```python
from build123d import *

# Parameters (mm, degrees)
F0_W          = 20
F0_H          = 20
F1_DEPTH      = 20
F3_R          = 2
F8_DEPTH      = 1
F2_R          = 2
F11_DEPTH     = 1
F6_R          = 2.787917168
F12_DEPTH     = 1
F4_R          = 2
F13_DEPTH     = 1
F14_DEPTH     = 1
F5_R          = 2
F15_DEPTH     = 1
F7_R          = 2
F16_DEPTH     = 1
F17_T1_DEPTH  = 16
F17_T3_DEPTH  = 16
F17_T5_DEPTH  = 16
F17_S9_W      = 2
F17_S9_H      = 2
F17_T10_DEPTH = 2
F17_S15_W     = 2
F17_S15_H     = 2
F17_T16_DEPTH = 2
F17_S21_W     = 2
F17_S21_H     = 2
F17_T22_DEPTH = 2
F17_S27_W     = 2
F17_S27_H     = 2
F17_T28_DEPTH = 2
F17_S33_W     = 2
F17_S33_H     = 2
F17_T34_DEPTH = 2
F17_S39_W     = 2
F17_S39_H     = 2
F17_T40_DEPTH = 2
F17_S45_W     = 2
F17_S45_H     = 2
F17_T46_DEPTH = 2
F17_S51_W     = 2
F17_S51_H     = 2
F17_T52_DEPTH = 2


# Not quite as in the source:
# - a fillet or chamfer that OpenCascade refuses, or shapes differently, is made with other operations: its cross-section is extruded or revolved along the edge and cut away or added
# - a feature of the source that left no trace in its solid (it failed there, or was rolled back) is left out


with BuildPart() as f1:
    # F0 (on Top) → F1 (new body)
    with BuildSketch(Plane.XY):
        with Locations((10, 10)):
            Rectangle(F0_W, F0_H)
    extrude(amount=F1_DEPTH)

    # F3 (on face) → F8 (cut)
    with BuildSketch(Plane.XY.offset(20)):
        with Locations((4.0282921307, 15.9717078693)):
            Circle(F3_R)
        with Locations((4.0282921307, 9.9717078693)):
            Circle(F3_R)
        with Locations((4.0282921307, 3.9717078693)):
            Circle(F3_R)
        with Locations((16.0282921307, 15.9717078693)):
            Circle(F3_R)
        with Locations((16.0282921307, 9.9717078693)):
            Circle(F3_R)
        with Locations((16.0282921307, 3.9717078693)):
            Circle(F3_R)
    extrude(amount=-F8_DEPTH, mode=Mode.SUBTRACT)

    # F2 (on Top) → F11 (cut)
    with BuildSketch(Plane.XY):
        with Locations((10, 10)):
            Circle(F2_R)
    extrude(amount=F11_DEPTH, mode=Mode.SUBTRACT)

    # F6 (on face) → F12 (cut)
    with BuildSketch(Plane(origin=(0, 0, 0), x_dir=(0, -1, 0), z_dir=(-1, 0, 0))):
        with Locations((-15.4005342424, 15.4005342424)):
            Circle(F6_R)
        with Locations((-10.667038206, 10.667038206)):
            Circle(F6_R)
        with Locations((-5.3520903582, 5.3520903582)):
            Circle(F6_R)
    extrude(amount=-F12_DEPTH, mode=Mode.SUBTRACT)

    # F4 (on Front) → F13 (cut)
    with BuildSketch(Plane.XZ):
        with Locations((16, 4)):
            Circle(F4_R)
        with Locations((4, 16)):
            Circle(F4_R)
        with Locations((16, 16)):
            Circle(F4_R)
        with Locations((4, 4)):
            Circle(F4_R)
        with Locations((10, 10)):
            Circle(F4_R)
    extrude(amount=-F13_DEPTH, mode=Mode.SUBTRACT)

    # F6 (on face) → F14 (cut)
    with BuildSketch(Plane(origin=(0, 0, 0), x_dir=(0, -1, 0), z_dir=(-1, 0, 0))):
        with Locations((-15.4005342424, 15.4005342424)):
            Circle(F6_R)
        with Locations((-10.667038206, 10.667038206)):
            Circle(F6_R)
        with Locations((-5.3520903582, 5.3520903582)):
            Circle(F6_R)
    extrude(amount=-F14_DEPTH, mode=Mode.SUBTRACT)

    # F5 (on face) → F15 (cut)
    with BuildSketch(Plane(origin=(0, 20, 0), x_dir=(-1, 0, 0), z_dir=(0, 1, 0))):
        with Locations((-13.3333333333, 13.3333333333)):
            Circle(F5_R)
        with Locations((-6.6666666667, 6.6666666667)):
            Circle(F5_R)
    extrude(amount=-F15_DEPTH, mode=Mode.SUBTRACT)

    # F7 (on face) → F16 (cut)
    with BuildSketch(Plane.YZ.offset(20)):
        with Locations((16, 4)):
            Circle(F7_R)
        with Locations((16, 16)):
            Circle(F7_R)
        with Locations((4, 16)):
            Circle(F7_R)
        with Locations((4, 4)):
            Circle(F7_R)
    extrude(amount=-F16_DEPTH, mode=Mode.SUBTRACT)

    # F17: fillet of radius 2 on 12 edges, made by hand

    # F17_s2 → F17_t1 (cut)
    with BuildSketch(Plane.YZ.offset(2)):
        with BuildLine():
            ThreePointArc((20, 2), (19.4142135624, 0.5857864376), (18, 0))
            Line((18, 0), (20, 0))
            Line((20, 0), (20, 2))
        make_face()
        with BuildLine():
            ThreePointArc((2, 0), (0.5857864376, 0.5857864376), (0, 2))
            Line((0, 2), (0, 0))
            Line((0, 0), (2, 0))
        make_face()
        with BuildLine():
            ThreePointArc((2, 20), (0.5857864376, 19.4142135624), (0, 18))
            Line((0, 18), (0, 20))
            Line((0, 20), (2, 20))
        make_face()
        with BuildLine():
            ThreePointArc((20, 18), (19.4142135624, 19.4142135624), (18, 20))
            Line((18, 20), (20, 20))
            Line((20, 20), (20, 18))
        make_face()
    extrude(amount=F17_T1_DEPTH, mode=Mode.SUBTRACT)

    # F17_s4 → F17_t3 (cut)
    with BuildSketch(Plane.XZ.offset(-18)):
        with BuildLine():
            ThreePointArc((18, 0), (19.4142135624, 0.5857864376), (20, 2))
            Line((20, 2), (20, 0))
            Line((20, 0), (18, 0))
        make_face()
        with BuildLine():
            ThreePointArc((0, 2), (0.5857864376, 0.5857864376), (2, 0))
            Line((2, 0), (0, 0))
            Line((0, 0), (0, 2))
        make_face()
        with BuildLine():
            ThreePointArc((0, 18), (0.5857864376, 19.4142135624), (2, 20))
            Line((2, 20), (0, 20))
            Line((0, 20), (0, 18))
        make_face()
        with BuildLine():
            ThreePointArc((18, 20), (19.4142135624, 19.4142135624), (20, 18))
            Line((20, 18), (20, 20))
            Line((20, 20), (18, 20))
        make_face()
    extrude(amount=F17_T3_DEPTH, mode=Mode.SUBTRACT)

    # F17_s6 → F17_t5 (cut)
    with BuildSketch(Plane.XY.offset(2)):
        with BuildLine():
            ThreePointArc((0, 2), (0.5857864376, 0.5857864376), (2, 0))
            Line((2, 0), (0, 0))
            Line((0, 0), (0, 2))
        make_face()
        with BuildLine():
            ThreePointArc((0, 18), (0.5857864376, 19.4142135624), (2, 20))
            Line((2, 20), (0, 20))
            Line((0, 20), (0, 18))
        make_face()
        with BuildLine():
            ThreePointArc((18, 0), (19.4142135624, 0.5857864376), (20, 2))
            Line((20, 2), (20, 0))
            Line((20, 0), (18, 0))
        make_face()
        with BuildLine():
            ThreePointArc((18, 20), (19.4142135624, 19.4142135624), (20, 18))
            Line((20, 18), (20, 20))
            Line((20, 20), (18, 20))
        make_face()
    extrude(amount=F17_T5_DEPTH, mode=Mode.SUBTRACT)


with BuildPart() as f17_tool8:
    # F17_s9 → F17_t10 (new body)
    with BuildSketch(Plane.YZ.offset(18)):
        with Locations((19, 1)):
            Rectangle(F17_S9_W, F17_S9_H)
    extrude(amount=F17_T10_DEPTH)

    # F17_s11 → F17_t12 (revolve, cut)
    with BuildSketch(Plane(origin=(18, 18, 2), x_dir=(0, -0.7071067812, 0.7071067812), z_dir=(0, 0.7071067812, 0.7071067812))):
        with BuildLine():
            ThreePointArc((0, -2), (2, 0), (0, 2))
            Line((0, 2), (0, -2))
        make_face()
    revolve(axis=Axis((18, 18, 2), (1, 0, 0)), mode=Mode.SUBTRACT)


with BuildPart() as f1_1:
    add(f1.part)

    # F17_t7: cut F17_tool8
    add(f17_tool8.part, mode=Mode.SUBTRACT)


with BuildPart() as f17_tool14:
    # F17_s15 → F17_t16 (new body)
    with BuildSketch(Plane.YZ.offset(2)):
        with Locations((19, 1)):
            Rectangle(F17_S15_W, F17_S15_H)
    extrude(amount=-F17_T16_DEPTH)

    # F17_s17 → F17_t18 (revolve, cut)
    with BuildSketch(Plane(origin=(2, 18, 2), x_dir=(0, -0.7071067812, 0.7071067812), z_dir=(0, -0.7071067812, -0.7071067812))):
        with BuildLine():
            ThreePointArc((0, -2), (2, 0), (0, 2))
            Line((0, 2), (0, -2))
        make_face()
    revolve(axis=Axis((2, 18, 2), (-1, 0, 0)), mode=Mode.SUBTRACT)


with BuildPart() as f1_2:
    add(f1_1.part)

    # F17_t13: cut F17_tool14
    add(f17_tool14.part, mode=Mode.SUBTRACT)


with BuildPart() as f17_tool20:
    # F17_s21 → F17_t22 (new body)
    with BuildSketch(Plane.YZ.offset(18)):
        with Locations((1, 1)):
            Rectangle(F17_S21_W, F17_S21_H)
    extrude(amount=F17_T22_DEPTH)

    # F17_s23 → F17_t24 (revolve, cut)
    with BuildSketch(Plane(origin=(18, 2, 2), x_dir=(0, 0.7071067812, 0.7071067812), z_dir=(0, 0.7071067812, -0.7071067812))):
        with BuildLine():
            ThreePointArc((0, -2), (2, 0), (0, 2))
            Line((0, 2), (0, -2))
        make_face()
    revolve(axis=Axis((18, 2, 2), (1, 0, 0)), mode=Mode.SUBTRACT)


with BuildPart() as f1_3:
    add(f1_2.part)

    # F17_t19: cut F17_tool20
    add(f17_tool20.part, mode=Mode.SUBTRACT)


with BuildPart() as f17_tool26:
    # F17_s27 → F17_t28 (new body)
    with BuildSketch(Plane.YZ.offset(2)):
        with Locations((1, 1)):
            Rectangle(F17_S27_W, F17_S27_H)
    extrude(amount=-F17_T28_DEPTH)

    # F17_s29 → F17_t30 (revolve, cut)
    with BuildSketch(Plane(origin=(2, 2, 2), x_dir=(0, 0.7071067812, 0.7071067812), z_dir=(0, -0.7071067812, 0.7071067812))):
        with BuildLine():
            ThreePointArc((0, -2), (2, 0), (0, 2))
            Line((0, 2), (0, -2))
        make_face()
    revolve(axis=Axis((2, 2, 2), (-1, 0, 0)), mode=Mode.SUBTRACT)


with BuildPart() as f1_4:
    add(f1_3.part)

    # F17_t25: cut F17_tool26
    add(f17_tool26.part, mode=Mode.SUBTRACT)


with BuildPart() as f17_tool32:
    # F17_s33 → F17_t34 (new body)
    with BuildSketch(Plane.YZ.offset(2)):
        with Locations((1, 19)):
            Rectangle(F17_S33_W, F17_S33_H)
    extrude(amount=-F17_T34_DEPTH)

    # F17_s35 → F17_t36 (revolve, cut)
    with BuildSketch(Plane(origin=(2, 2, 18), x_dir=(0, 0.7071067812, -0.7071067812), z_dir=(0, 0.7071067812, 0.7071067812))):
        with BuildLine():
            ThreePointArc((0, -2), (2, 0), (0, 2))
            Line((0, 2), (0, -2))
        make_face()
    revolve(axis=Axis((2, 2, 18), (-1, 0, 0)), mode=Mode.SUBTRACT)


with BuildPart() as f1_5:
    add(f1_4.part)

    # F17_t31: cut F17_tool32
    add(f17_tool32.part, mode=Mode.SUBTRACT)


with BuildPart() as f17_tool38:
    # F17_s39 → F17_t40 (new body)
    with BuildSketch(Plane.YZ.offset(2)):
        with Locations((19, 19)):
            Rectangle(F17_S39_W, F17_S39_H)
    extrude(amount=-F17_T40_DEPTH)

    # F17_s41 → F17_t42 (revolve, cut)
    with BuildSketch(Plane(origin=(2, 18, 18), x_dir=(0, -0.7071067812, -0.7071067812), z_dir=(0, 0.7071067812, -0.7071067812))):
        with BuildLine():
            ThreePointArc((0, -2), (2, 0), (0, 2))
            Line((0, 2), (0, -2))
        make_face()
    revolve(axis=Axis((2, 18, 18), (-1, 0, 0)), mode=Mode.SUBTRACT)


with BuildPart() as f1_6:
    add(f1_5.part)

    # F17_t37: cut F17_tool38
    add(f17_tool38.part, mode=Mode.SUBTRACT)


with BuildPart() as f17_tool44:
    # F17_s45 → F17_t46 (new body)
    with BuildSketch(Plane.YZ.offset(18)):
        with Locations((1, 19)):
            Rectangle(F17_S45_W, F17_S45_H)
    extrude(amount=F17_T46_DEPTH)

    # F17_s47 → F17_t48 (revolve, cut)
    with BuildSketch(Plane(origin=(18, 2, 18), x_dir=(0, 0.7071067812, -0.7071067812), z_dir=(0, -0.7071067812, -0.7071067812))):
        with BuildLine():
            ThreePointArc((0, -2), (2, 0), (0, 2))
            Line((0, 2), (0, -2))
        make_face()
    revolve(axis=Axis((18, 2, 18), (1, 0, 0)), mode=Mode.SUBTRACT)


with BuildPart() as f1_7:
    add(f1_6.part)

    # F17_t43: cut F17_tool44
    add(f17_tool44.part, mode=Mode.SUBTRACT)


with BuildPart() as f17_tool50:
    # F17_s51 → F17_t52 (new body)
    with BuildSketch(Plane.YZ.offset(18)):
        with Locations((19, 19)):
            Rectangle(F17_S51_W, F17_S51_H)
    extrude(amount=F17_T52_DEPTH)

    # F17_s53 → F17_t54 (revolve, cut)
    with BuildSketch(Plane(origin=(18, 18, 18), x_dir=(0, -0.7071067812, -0.7071067812), z_dir=(0, -0.7071067812, 0.7071067812))):
        with BuildLine():
            ThreePointArc((0, -2), (2, 0), (0, 2))
            Line((0, 2), (0, -2))
        make_face()
    revolve(axis=Axis((18, 18, 18), (1, 0, 0)), mode=Mode.SUBTRACT)


with BuildPart() as f1_8:
    add(f1_7.part)

    # F17_t49: cut F17_tool50
    add(f17_tool50.part, mode=Mode.SUBTRACT)


solid = f1_8.part
```
CAD build for the part. Positions are in the model's coordinates, mm. A direction names the side the tool comes from. Round coordinates to 2 decimals unless told otherwise and drop trailing zeros. Order: outer loops, then holes, each group sorted by start corner. A loop starts at its lowest first (then second) coordinate and runs counter-clockwise, first axis right, second up.
Q1. Slice it at A-A (x = 10). Write the cut outline in (y, z), and give its area (3 significant figures).
Q2. Slice it at C-C (z = 10). Write the cut outline in (x, y).
Q3. Drop a flat-ended pin along its axis: pin 1 (1.2 mm diameter, centred on x = 13, z = 12.5, fed in from +Y). Give the stop position or say it passes through.
Q4. Slice it at B-B (y = 11.25). Write the cut outline in (x, z).
Q5. Which spindle directions (+Z, -Z, +X, -X, +Y, -Y) get a long thin tool onto all of the face, cutting with end or side? Do faces 1 (the flat face through (1, 15, 15)), 2 (the cylindrical face through (4.951, 2.197, 19.507)), 3 (the cylindrical face through (9.74, 0.493, 11.983)). Say none if no direction does.
Q6. Slice it at D-D (y = 15.25). Write the cut outline in (x, z), and give its area (3 significant figures).
Q7. Wall check: L1, parallel to Z at x = 19.3, y = 16; L2, parallel to Y at x = 17.25, z = 3; L3, parallel to Z at x = 16, y = 14.5. Give the ranges that are in metal, low to high.
Q8. Two-plate mould, pull along Z, no slides. Class faces 4 (the cylindrical face through (0.57, 10.11, 0.6)), 5 (the cylindrical face through (19.507, 15.74, 17.983)), 6 (the cylindrical face through (9.89, 19.43, 19.4)): pulls with the +Z half, pulls with the -Z half, needs draft (parallel to the pull), parting line crosses it, or undercut.
Results below:
1. outline: (0, 2) arc R2 ccw to (2, 0) - (8, 0) - (8, 1) - (12, 1) - (12, 0) - (18, 0) arc R2 ccw to (20, 2) - (20, 18) arc R2 ccw to (18, 20) - (2, 20) arc R2 ccw to (0, 18) - (0, 12) - (1, 12) - (1, 8) - (0, 8) - close
1. area: 389 mm2
2. outline: (0, 2) arc R2 ccw to (2, 0) - (8, 0) - (8, 1) - (12, 1) - (12, 0) - (18, 0) arc R2 ccw to (20, 2) - (20, 18) arc R2 ccw to (18, 20) - (2, 20) arc R2 ccw to (0, 18) - (0, 13.37) - (1, 13.37) - (1, 7.96) - (0, 7.96) - close
3. pin 1: stops at y = 19
4. outline: (0, 2) arc R2 ccw to (2, 0) - (8.44, 0) - (8.44, 1) - (11.56, 1) - (11.56, 0) - (18, 0) arc R2 ccw to (20, 2) - (20, 18) arc R2 ccw to (18, 20) - (17.57, 20) - (17.57, 19) - (14.49, 19) - (14.49, 20) - (5.57, 20) - (5.57, 19) - (2.49, 19) - (2.49, 20) - (2, 20) arc R2 ccw to (0, 18) - (0, 13.39) - (1, 13.39) - (1, 7.94) - (0, 7.94) - close
5. face 1: -X
5. face 2: +Z
5. face 3: -Y
6. outline: (0, 2) arc R2 ccw to (2, 0) - (18, 0) arc R2 ccw to (20, 2) - (20, 2.15) - (19, 2.15) - (19, 5.85) - (20, 5.85) - (20, 14.15) - (19, 14.15) - (19, 17.85) - (20, 17.85) - (20, 18) arc R2 ccw to (18, 20) - (17.89, 20) - (17.89, 19) - (14.16, 19) - (14.16, 20) - (5.89, 20) - (5.89, 19) - (2.16, 19) - (2.16, 20) - (2, 20) arc R2 ccw to (0.01, 18.18) - (1, 18.18) - (1, 12.62) - (0, 12.62) - close
6. area: 376 mm2
7. L1: z = 0.48 to 2, 6 to 14, 18 to 19.52
7. L2: y = 1 to 20
7. L3: z = 0 to 19
8. face 4: pulls with the -Z half
8. face 5: undercut
8. face 6: pulls with the +Z half
